Could you check a few things on this model? Use its own coordinates, in mm. A direction names the side the tool comes from. Coordinates: 2 decimals unless noted, no trailing zeros. Write each loop counter-clockwise with the first axis right and the second up, starting at its lowest first coordinate (ties: lowest second). Pieces come first, ordered by that corner, then holes. Notation, with made-up numbers: M 68,81.25 L 108,81.25 A17 cw 108,111.25 Z; hole C -29,73.5 d8. An arc over 180 degrees is marked long. Write item = value, one per line.
```python
from build123d import *

# Parameters (mm, degrees)
SKETCH1_R           = 7.5
BOSS_EXTRUDE1_DEPTH = 20
BOSS_EXTRUDE2_DEPTH = 6
SKETCH3_R           = 4.5
CUT_EXTRUDE1_DEPTH  = 24.58495283


with BuildPart() as part:
    # Sketch1 → Boss-Extrude1 (new body)
    with BuildSketch(Plane.XY):
        Circle(SKETCH1_R)
    extrude(amount=BOSS_EXTRUDE1_DEPTH)

    # Sketch2 → Boss-Extrude2 (add)
    with BuildSketch(Plane(origin=(0, 0, 0), x_dir=(-1, 0, 0), z_dir=(0, 0, -1))):
        with BuildLine():
            Line((2.75, -9.614442262), (2.75, 9.614442262))
            ThreePointArc((2.75, 9.614442262), (0, 10), (-2.75, 9.614442262))
            Line((-2.75, 9.614442262), (-2.75, -9.614442262))
            ThreePointArc((-2.75, -9.614442262), (0, -10), (2.75, -9.614442262))
        make_face()
    extrude(amount=-BOSS_EXTRUDE2_DEPTH)

    # Sketch3 → Cut-Extrude1 (cut, through all)
    with BuildSketch(Plane(origin=(0, 0, 0), x_dir=(-1, 0, 0), z_dir=(0, 0, -1))):
        Circle(SKETCH3_R)
    extrude(amount=-CUT_EXTRUDE1_DEPTH, mode=Mode.SUBTRACT)


solid = part.part
```
Item 1: I'm going to push flat-ended pins straight in: P1, Ø3, axis at y = -8, z = 3, coming from the -X side; P2, Ø8, axis at y = -1.5, z = 17, coming from the +X side; P3, Ø6, axis at y = -3.5, z = 4.5, coming from the -X side; P4, Ø10, axis at y = 8, z = 12, coming from the -X side. Where does each tip first touch, or does it pass through?
Numbers:
P1 = -3.74
P2 = 7.5
P3 = -7.48
P4 = -6.87
Item 2: For faces 4 (the face through (2.75, -8, 3)), 5 (the face through (7.154, 2.253, 9.86)), 6 (the face through (-2.75, -8, 3)), which set-ups out of +Z, -Z, +X, -X, +Y, -Y let a thin tool reach every point of the face, with its end or its side?
Numbers:
face_4 = +Z, -Z, +X, -Y
face_5 = +Z
face_6 = +Z, -Z, -X, -Y
Item 3: Imagine slicing it at D-D (y = -3.5). Write out the boundary of the cut face in (x, z), and give its area (3 significant figures).
Numbers:
outline = M -6.63,0 L -2.83,0 L -2.83,20 L -6.63,20 Z; M 2.83,0 L 6.63,0 L 6.63,20 L 2.83,20 Z
area = 152 mm²
Item 4: If I drill on line 1 along Y through (x, z) = (0, 5.5); line 2 along Y through (x, z) = (0, 11); line 3 along Z through (x, y) = (-2.5, -7.5), over which ranges is the centre line in solid material (lowest first)?
Numbers:
line_1 = -10 to -4.5, 4.5 to 10
line_2 = -7.5 to -4.5, 4.5 to 7.5
line_3 = 0 to 6
Item 5: If we mould it in two halves opening along Y, with no side actions, what happens to faces 1 (the face through (0, -8, 6)), 2 (the face through (0.59, 4.46, 9.86)), 3 (the face through (0, -10, 3))? For each: pulls with the +Y half, pulls with the -Y half, needs draft (parallel to the pull), parting line crosses it, or undercut.
Numbers:
face_1 = needs draft
face_2 = undercut
face_3 = pulls with the -Y half
Item 6: Imagine slicing it at A-A (x = 0). Write out the boundary of the cut face in (y, z).
Numbers:
outline = M -10,0 L -4.5,0 L -4.5,20 L -7.5,20 L -7.5,6 L -10,6 Z; M 4.5,0 L 10,0 L 10,6 L 7.5,6 L 7.5,20 L 4.5,20 Z
Item 7: Imagine slicing it at B-B (y = 0). Write out the boundary of the cut face in (x, z), and give its area (3 significant figures).
Numbers:
outline = M -7.5,0 L -4.5,0 L -4.5,20 L -7.5,20 Z; M 4.5,0 L 7.5,0 L 7.5,20 L 4.5,20 Z
area = 120 mm²
Item 8: Imagine slicing it at C-C (z = 12.75). Write out the boundary of the cut face in (x, y).
Numbers:
outline = C 0,0 d15; hole C 0,0 d9
